Geometry check sheet. Reference: the model listing, model coordinates, mm. A direction names the side the tool comes from. Round coordinates to 2 decimals unless told otherwise and drop trailing zeros. Write each loop counter-clockwise with the first axis right and the second up, starting at its lowest first coordinate (ties: lowest second). Pieces come first, ordered by that corner, then holes.
Item 1: Cross-section at B-B (x = 31.5). Enter the section's corners in (y, z) (3 decimals).
Item 2: Cross-section at D-D (y = 38.1). Enter the section's corners in (x, z), then the cut area to 3 significant figures.
Item 3: Scan lines: probe 1 along X at (y, z) = (63.5, -2.2); probe 2 along Y at (x, z) = (1.6, -15.7); probe 3 along Z at (x, y) = (21.5, 35.5). Record each from-to range of solid material in increasing order.
Item 4: Depth check by flat-ended pin: P1, Ø12, axis at x = 28, z = -26.5, coming from the -Y side; P2, Ø1.9, axis at x = 2.5, z = -21, coming from the +Y side; P3, Ø6.5, axis at y = 38.1, z = -15.7, coming from the +X side. Enter the tip coordinate at first touch or a pass-through.
Item 5: Draft check along Y on faces 1 (the face through (1.48, 27.87, -16.02)), 2 (the face through (9.569, 69.894, -1.479)), 3 (the face through (36.59, 61.52, -29.92)), 4 (the face through (25, 44, -28.4)). Enter one of: pulls with the +Y half, pulls with the -Y half, needs draft (parallel to the pull), parting line crosses it, or undercut.
Item 6: Cross-section at A-A (y = 56.5). Enter the section's corners in (x, z).
Item 7: Access from +Z, -Z, +X, -X, +Y, -Y to the whole of each face (thin tool, end or side, straight path). Record for faces 5 (the face through (1.479, 35.892, -14.551)), 6 (the face through (3, 26, -13)).
Item 8: Cross-section at C-C (x = 49.5). Enter the section's corners in (y, z) (3 decimals).
from build123d import *

# Parameters (mm, degrees)
SKETCH7_W                  = 50.8
SKETCH7_H                  = 24.1808
BASE_FLANGE1_DEPTH         = 3
F_9_0_196_DIAMETER_HOLE1_D = 4.9784
EDGE_FLANGE1_DEPTH         = 50.8
EDGE_FLANGE1_START         = 3
EDGE_FLANGE1_PROFILE_R     = 2.4892
EDGE_FLANGE1_FLAT_DEPTH    = 3
EDGE_FLANGE2_DEPTH         = 50.8
EDGE_FLANGE2_START         = 3
EDGE_FLANGE2_PROFILE_R     = 2.4892
EDGE_FLANGE2_FLAT_DEPTH    = 3


# Sheet-metal steps are written as plain solids
with BuildPart() as part:
    # Sketch7 → Base-Flange1 (new body)
    with BuildSketch(Plane(origin=(0, 0, 0), x_dir=(0, -1, 0), z_dir=(-1, 0, 0))):
        with Locations((-25.4, -15.7)):
            Rectangle(SKETCH7_W, SKETCH7_H)
    extrude(amount=-BASE_FLANGE1_DEPTH)

    # #9 (0.196) Diameter Hole1 (through all)
    with Locations(Plane(origin=(3, 0, 0), x_dir=(0, 0, -1), z_dir=(1, 0, 0))):
        with Locations((15.7, 25.4), (15.7, 12.7), (15.7, 38.1)):
            Hole(F_9_0_196_DIAMETER_HOLE1_D / 2)

    # Edge-Flange1 bend section (across the edge) → Edge-Flange1 (add)
    with BuildSketch(Plane(origin=(3, 0, -28.4), x_dir=(0, 0, 1), z_dir=(0, 1, 0))):
        with BuildLine():
            Line((-3, 0.6096), (0, 0.6096))
            ThreePointArc((0, 0.6096), (0.178547706, 0.178547706), (0.6096, 0))
            Line((0.6096, 0), (0.6096, -3))
            ThreePointArc((0.6096, -3), (-1.942772637, -1.942772637), (-3, 0.6096))
        make_face()
    extrude(amount=EDGE_FLANGE1_DEPTH)

    # Edge-Flange1 profile (on flange) → Edge-Flange1 flat (add)
    with BuildSketch(Plane(origin=(3, 0, -28.4), x_dir=(0, 1, 0), z_dir=(0, 0, -1)).offset(EDGE_FLANGE1_START)):
        Polygon((0, 0.6096), (50.8, 0.6096), (50.8, 3.35), (66.675, 3.35), (73.025, 9.7), (73.025, 47.8), (66.675, 54.15), (50.8, 54.15), (0, 9.7), align=None)
        with Locations((63.5, 9.7)):
            Circle(EDGE_FLANGE1_PROFILE_R, mode=Mode.SUBTRACT)
        with Locations((63.5, 22.4)):
            Circle(EDGE_FLANGE1_PROFILE_R, mode=Mode.SUBTRACT)
        with Locations((63.5, 35.1)):
            Circle(EDGE_FLANGE1_PROFILE_R, mode=Mode.SUBTRACT)
        with Locations((63.5, 47.8)):
            Circle(EDGE_FLANGE1_PROFILE_R, mode=Mode.SUBTRACT)
    extrude(amount=-EDGE_FLANGE1_FLAT_DEPTH)

    # Edge-Flange2 bend section (across the edge) → Edge-Flange2 (add)
    with BuildSketch(Plane(origin=(3, 50.8, -3), x_dir=(0, 0, -1), z_dir=(0, -1, 0))):
        with BuildLine():
            Line((-3, 0.6096), (0, 0.6096))
            ThreePointArc((0, 0.6096), (0.178547706, 0.178547706), (0.6096, 0))
            Line((0.6096, 0), (0.6096, -3))
            ThreePointArc((0.6096, -3), (-1.942772637, -1.942772637), (-3, 0.6096))
        make_face()
    extrude(amount=EDGE_FLANGE2_DEPTH)

    # Edge-Flange2 profile (on flange) → Edge-Flange2 flat (add)
    with BuildSketch(Plane(origin=(3, 0, -3), x_dir=(0, -1, 0), z_dir=(0, 0, 1)).offset(EDGE_FLANGE2_START)):
        Polygon((0, 0.6096), (0, 9.7), (-50.8, 54.15), (-66.675, 54.15), (-73.025, 47.8), (-73.025, 9.7), (-66.675, 3.35), (-50.8, 3.35), (-50.8, 0.6096), align=None)
        with Locations((-63.5, 9.7)):
            Circle(EDGE_FLANGE2_PROFILE_R, mode=Mode.SUBTRACT)
        with Locations((-63.5, 22.4)):
            Circle(EDGE_FLANGE2_PROFILE_R, mode=Mode.SUBTRACT)
        with Locations((-63.5, 35.1)):
            Circle(EDGE_FLANGE2_PROFILE_R, mode=Mode.SUBTRACT)
        with Locations((-63.5, 47.8)):
            Circle(EDGE_FLANGE2_PROFILE_R, mode=Mode.SUBTRACT)
    extrude(amount=-EDGE_FLANGE2_FLAT_DEPTH)


solid = part.part
Resolved:
1. outline: (21.486, -31.4) - (73.025, -31.4) - (73.025, -28.4) - (21.486, -28.4) - close; (21.486, -3) - (73.025, -3) - (73.025, 0) - (21.486, 0) - close
2. outline: (0, -27.79) arc R3.61 ccw to (3.61, -31.4) - (46.04, -31.4) - (46.04, -28.4) - (3.61, -28.4) arc R0.61 cw to (3, -27.79) - (3, -18.19) - (0, -18.19) - close; (0, -13.21) - (3, -13.21) - (3, -3.61) arc R0.61 cw to (3.61, -3) - (46.04, -3) - (46.04, 0) - (3.61, 0) arc R3.61 ccw to (0, -3.61) - close
2. area: 332 mm2
3. probe 1: x = 6.35 to 10.21, 15.19 to 22.91, 27.89 to 35.61, 40.59 to 48.31, 53.29 to 57.15
3. probe 2: y = 0 to 10.21, 15.19 to 22.91, 27.89 to 35.61, 40.59 to 50.8
3. probe 3: z = -31.4 to -28.4, -3 to 0
4. P1: stops at y = 10.98
4. P2: stops at y = 50.8
4. P3: stops at x = 3
5. face 1: undercut
5. face 2: pulls with the +Y half
5. face 3: undercut
5. face 4: needs draft
6. outline: (6.35, -31.4) - (57.15, -31.4) - (57.15, -28.4) - (6.35, -28.4) - close; (6.35, -3) - (57.15, -3) - (57.15, 0) - (6.35, 0) - close
7. face 5: +X, -X
7. face 6: +X, +Y, -Y
8. outline: (42.057, -31.4) - (61.377, -31.4) - (61.377, -28.4) - (42.057, -28.4) - close; (42.057, -3) - (61.377, -3) - (61.377, 0) - (42.057, 0) - close; (65.623, -31.4) - (73.025, -31.4) - (73.025, -28.4) - (65.623, -28.4) - close; (65.623, -3) - (73.025, -3) - (73.025, 0) - (65.623, 0) - close
